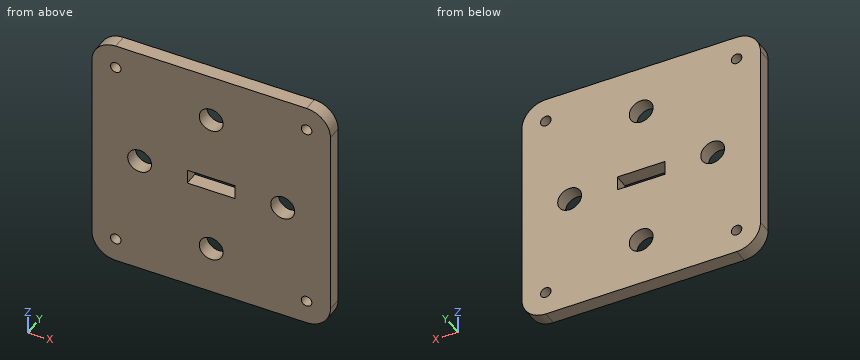
```python
from build123d import *

# Parameters (mm, degrees)
SKETCH1_W           = 50
SKETCH1_H           = 50
SKETCH1_R           = 2.5
SKETCH1_R_2         = 1.1
SKETCH1_W_2         = 10
SKETCH1_H_2         = 3
BOSS_EXTRUDE1_DEPTH = 3
FILLET1_R           = 5


with BuildPart() as part:
    # Sketch1 → Boss-Extrude1 (new body)
    with BuildSketch(Plane(origin=(0, 0, 0), x_dir=(1, 0, 0), z_dir=(0, 1, 0))):
        Rectangle(SKETCH1_W, SKETCH1_H)
        with Locations(Location((-15, 0, 0), (0, 0, 270))):
            Circle(SKETCH1_R, mode=Mode.SUBTRACT)
        with Locations(Location((15, 0, 0), (0, 0, 90))):
            Circle(SKETCH1_R, mode=Mode.SUBTRACT)
        with Locations(Location((-20, 20, 0), (0, 0, 270))):
            Circle(SKETCH1_R_2, mode=Mode.SUBTRACT)
        with Locations(Location((20, 20, 0), (0, 0, 90))):
            Circle(SKETCH1_R_2, mode=Mode.SUBTRACT)
        with Locations(Location((20, -20, 0), (0, 0, 270))):
            Circle(SKETCH1_R_2, mode=Mode.SUBTRACT)
        with Locations(Location((-20, -20, 0), (0, 0, 90))):
            Circle(SKETCH1_R_2, mode=Mode.SUBTRACT)
        with Locations(Location((0, 15, 0), (0, 0, 270))):
            Circle(SKETCH1_R, mode=Mode.SUBTRACT)
        with Locations(Location((0, -15, 0), (0, 0, 90))):
            Circle(SKETCH1_R, mode=Mode.SUBTRACT)
        Rectangle(SKETCH1_W_2, SKETCH1_H_2, mode=Mode.SUBTRACT)
    extrude(amount=BOSS_EXTRUDE1_DEPTH)

    # Fillet1
    fillet1_edges = [part.edges().sort_by_distance(p)[0] for p in [
        (25, 1.5, 25),
        (-25, 1.5, 25),
        (-25, 1.5, -25),
        (25, 1.5, -25),
    ]]
    fillet(fillet1_edges, radius=FILLET1_R)


solid = part.part
```
Geometry: final body of the model. Coordinates: model frame, mm. Round coordinates to 2 decimals unless told otherwise and drop trailing zeros. Order: outer loops, then holes, each group sorted by start corner. A loop starts at its lowest first (then second) coordinate and runs counter-clockwise, first axis right, second up. Notation, with made-up numbers: M 75,27.5 L 109,27.5 A20 ccw 109,32.5 Z; hole C -1.5,62.5 d10. An arc over 180 degrees is marked long. Use one line per item in the form item = value. Start each with the question number.
Q1. Cut plane D-D (x = -22). Return loops of the section in (y, z).
Q2. Cut plane A-A (x = 15). Return loops of the section in (y, z), and give its area (3 significant figures).
Q3. Material intervals for line 1 (X direction, y = 1.45, z = 20); line 2 (Z direction, x = 15, y = 2.05); line 3 (Z direction, x = 3.5, y = 2.4), sorted ascending. Write a range as [from, to].
Q4. Cut plane B-B (z = 15). Return loops of the section in (x, y).
Q5. Cut plane C-C (y = 1.25). Count the separate pieces of the cut face and the enclosed holes in it, and give its area (3 significant figures).
Geometry results:
q1.outline = M 0,-24.58 L 3,-24.58 L 3,24.58 L 0,24.58 Z
q2.outline = M 0,-25 L 3,-25 L 3,-2.5 L 0,-2.5 Z; M 0,2.5 L 3,2.5 L 3,25 L 0,25 Z
q2.area = 135 mm^2
q3.line_1 = [-25, -21.1], [-18.9, 18.9], [21.1, 25]
q3.line_2 = [-25, -2.5], [2.5, 25]
q3.line_3 = [-25, -1.5], [1.5, 25]
q4.outline = M -25,0 L -2.5,0 L -2.5,3 L -25,3 Z; M 2.5,0 L 25,0 L 25,3 L 2.5,3 Z
q5.separate_pieces = 1
q5.enclosed_holes = 9
q5.area = 2,350 mm^2
